from build123d import *

# Parameters (mm, degrees)
CROQUIS1_R              = 4
SALIENTE_EXTRUIR1_DEPTH = 10


with BuildPart() as part:
    # Croquis1 → Saliente-Extruir1 (new body)
    with BuildSketch(Plane.XY):
        with BuildLine():
            ThreePointArc((-29.650108804, -13.308683176), (-27.580638973, -8.961492837), (-31.810089606, -6.660945822))
            ThreePointArc((-31.810089606, -6.660945822), (-32.5, 0), (-31.810089606, 6.660945822))
            ThreePointArc((-31.810089606, 6.660945822), (-27.580638973, 8.961492837), (-29.650108804, 13.308683176))
            ThreePointArc((-29.650108804, 13.308683176), (-26.293052317, 19.1030207), (-21.819697364, 24.086319913))
            ThreePointArc((-21.819697364, 24.086319913), (-17.045772316, 23.461492837), (-16.16479421, 28.194847546))
            ThreePointArc((-16.16479421, 28.194847546), (-10.043052317, 30.90933678), (-3.494922352, 32.311538462))
            ThreePointArc((-3.494922352, 32.311538462), (0, 29), (3.494922352, 32.311538462))
            ThreePointArc((3.494922352, 32.311538462), (10.043052317, 30.90933678), (16.16479421, 28.194847546))
            ThreePointArc((16.16479421, 28.194847546), (17.045772316, 23.461492837), (21.819697364, 24.086319913))
            ThreePointArc((21.819697364, 24.086319913), (26.293052317, 19.1030207), (29.650108804, 13.308683176))
            ThreePointArc((29.650108804, 13.308683176), (27.580638973, 8.961492837), (31.810089606, 6.660945822))
            ThreePointArc((31.810089606, 6.660945822), (32.5, 0), (31.810089606, -6.660945822))
            ThreePointArc((31.810089606, -6.660945822), (27.580638973, -8.961492837), (29.650108804, -13.308683176))
            ThreePointArc((29.650108804, -13.308683176), (26.293052317, -19.1030207), (21.819697364, -24.086319913))
            ThreePointArc((21.819697364, -24.086319913), (17.045772316, -23.461492837), (16.16479421, -28.194847546))
            ThreePointArc((16.16479421, -28.194847546), (10.043052317, -30.90933678), (3.494922352, -32.311538462))
            ThreePointArc((3.494922352, -32.311538462), (0, -29), (-3.494922352, -32.311538462))
            ThreePointArc((-3.494922352, -32.311538462), (-10.043052317, -30.90933678), (-16.16479421, -28.194847546))
            ThreePointArc((-16.16479421, -28.194847546), (-17.045772316, -23.461492837), (-21.819697364, -24.086319913))
            ThreePointArc((-21.819697364, -24.086319913), (-26.293052317, -19.1030207), (-29.650108804, -13.308683176))
        make_face()
        Circle(CROQUIS1_R, mode=Mode.SUBTRACT)
    extrude(amount=SALIENTE_EXTRUIR1_DEPTH)


solid = part.part
Work out the finished part from the listing and answer in its coordinate system (mm). Coordinates: 2 decimals unless noted, no trailing zeros. Write each loop counter-clockwise with the first axis right and the second up, starting at its lowest first coordinate (ties: lowest second). Pieces come first, ordered by that corner, then holes. Notation, with made-up numbers: M 89.5,-15 L 96.5,-15 A9 cw 96.5,0 Z; hole C 14.5,68.5 d11. An arc over 180 degrees is marked long. Answer as CSV lines item,"result". Start each with the question number.
Item 1: Section C-C on z = 1.75 is taken. Write down the section's boundary in (x, y), and give its area (3 significant figures).
Item 2: Flat-ended cylindrical pins translate along their axes: P1, Ø1, axis at y = 3.5, z = 3.5, coming from the +X side; P2, Ø2, axis at y = -5, z = 3.5, coming from the +X side; P3, Ø5, axis at y = -16.5, z = 6, coming from the +X side. Find the tip coordinate at first contact, or state that the pin passes through.
Item 3: Consider L1, parallel to X at y = 2, z = 7.25; L2, parallel to X at y = -1, z = 2.5; L3, parallel to X at y = -19, z = 3. Determine where each line is inside the solid, lowest interval first.
Item 4: Determine the mould class of faces 1 (the face through (0, 29, 5)), 2 (the face through (27.6, -8.9, 4.9)), 3 (the face through (10.13, -30.88, 4.93)), 4 (the face through (-26.348, 19.027, 4.93)) for opening direction X: released by +X, released by -X, zero draft, split by the parting line, or undercut.
Item 5: Section D-D on x = -19.5 is taken. Write down the section's boundary in (y, z), and give its area (3 significant figures).
Item 6: Section B-B on x = 0 is taken. Write down the section's boundary in (y, z), and give its area (3 significant figures).
Item 7: Section A-A on y = 0 is taken. Write down the section's boundary in (x, z).
Checks:
1,outline,"M -31.81,-6.66 A3.5 cw -29.65,-13.31 A32.5 ccw -21.82,-24.09 A3.5 cw -16.16,-28.19 A32.5 ccw -3.49,-32.31 A3.5 cw 3.49,-32.31 A32.5 ccw 16.16,-28.19 A3.5 cw 21.82,-24.09 A32.5 ccw 29.65,-13.31 A3.5 cw 31.81,-6.66 A32.5 ccw 31.81,6.66 A3.5 cw 29.65,13.31 A32.5 ccw 21.82,24.09 A3.5 cw 16.16,28.19 A32.5 ccw 3.49,32.31 A3.5 cw -3.49,32.31 A32.5 ccw -16.16,28.19 A3.5 cw -21.82,24.09 A32.5 ccw -29.65,13.31 A3.5 cw -31.81,6.66 A32.5 ccw Z; hole C 0,0 d8"
1,area,"3,080 mm²"
2,P1,"stops at x = 32.36"
2,P2,"stops at x = 32.25"
2,P3,"stops at x = 29.33"
3,L1,"x = -32.44 to -3.46, 3.46 to 32.44"
3,L2,"x = -32.48 to -3.87, 3.87 to 32.48"
3,L3,"x = -26.37 to 26.37"
4,face 1,"undercut"
4,face 2,"undercut"
4,face 3,"released by +X"
4,face 4,"released by -X"
5,outline,"M -22.82,0 L 22.82,0 L 22.82,10 L -22.82,10 Z"
5,area,"456 mm²"
6,outline,"M -29,0 L -4,0 L -4,10 L -29,10 Z; M 4,0 L 29,0 L 29,10 L 4,10 Z"
6,area,"500 mm²"
7,outline,"M -32.5,0 L -4,0 L -4,10 L -32.5,10 Z; M 4,0 L 32.5,0 L 32.5,10 L 4,10 Z"
